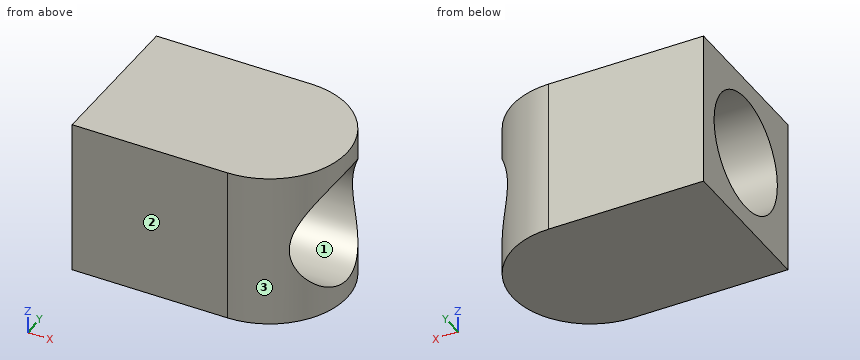
from build123d import *

# Parameters (mm, degrees)
SKETCH1_W           = 20
SKETCH1_H           = 20
BOSS_EXTRUDE1_DEPTH = 30
FILLET3_RADIUS      = 10
FILLET3_LENGTH      = 20
SKETCH2_R           = 7.5
CUT_EXTRUDE1_DEPTH  = 30


with BuildPart() as part:
    # Sketch1 → Boss-Extrude1 (new body)
    with BuildSketch(Plane(origin=(0, 0, 0), x_dir=(0, 0, -1), z_dir=(1, 0, 0))):
        Rectangle(SKETCH1_W, SKETCH1_H)
    extrude(amount=BOSS_EXTRUDE1_DEPTH)

    # Fillet3: full round fillet: the end face becomes a half cylinder, R = half its width
    fillet3_face = Plane((30, 0, 0), x_dir=(0, 0, 1), z_dir=(1, 0, 0))  # on the end face: x along it, z out of the body
    fillet3_slab = fillet3_face.offset(-FILLET3_RADIUS / 2) * Box(FILLET3_LENGTH, 2 * FILLET3_RADIUS, FILLET3_RADIUS, mode=Mode.PRIVATE)  # the body's end, R deep
    fillet3_round = Plane((20, 0, 0), x_dir=(1, 0, 0), z_dir=(0, 0, 1)) * Cylinder(FILLET3_RADIUS, FILLET3_LENGTH, mode=Mode.PRIVATE)  # its axis R under the face
    add(fillet3_slab - fillet3_round, mode=Mode.SUBTRACT)

    # Sketch2 → Cut-Extrude1 (cut)
    with BuildSketch(Plane.ZY):
        Circle(SKETCH2_R)
    extrude(amount=-CUT_EXTRUDE1_DEPTH, mode=Mode.SUBTRACT)


solid = part.part
Design review of the part built by this model. Coordinates are the model's own, in mm. Face numbers are marked on the shaded views. Coordinates: 2 decimals unless noted, no trailing zeros. Order: outer loops, then holes, each group sorted by start corner. A loop starts at its lowest first (then second) coordinate and runs counter-clockwise, first axis right, second up. Notation, with made-up numbers: (-26, -20.75) -> (2, -20.75) arc R9 cw to (2, -5.75) -> close; hole circle Ø8 at (-22.75, -12.75). An arc over 180 degrees is marked (long way). Use one line per item in the form item = value. Start each with the question number.
(1) For probe 1 along Y at (x, z) = (7.5, 0); probe 2 along Z at (x, y) = (17.5, -3.25), list the stretches that pass through material, from the lowest coordinate up.
(2) Add section C-C on x = 11. State the section outline as (y, z) points, plus the area to 3 significant figures.
(3) The part is to be moulded in two halves that separate along Y. For the marked faces 1, 2 and 3, say which applies: +Y half, -Y half, draft (parallel to the pull), parting line (faces both ways), or undercut.
(4) Add section D-D on z = 8. State the section outline as (x, y) points.
(5) Add section B-B on y = 0. State the section outline as (x, z) points.
(6) Add section A-A on z = -4.5. State the section outline as (x, y) points.
(7) Insertion check: pin 1 (10 mm diameter, centred on y = 7, z = -7.5, fed in from +X). The pin has a flat end and moves straight along its axis. Give the tip position at first contact, or say it passes through.
Answer block:
q1.probe_1 = -10 to -7.5, 7.5 to 10
q1.probe_2 = -10 to -6.76, 6.76 to 10
q2.outline = (-10, -10) -> (10, -10) -> (10, 10) -> (-10, 10) -> close; hole circle Ø15 at (0, 0)
q2.area = 223 mm²
q3.face_1 = undercut
q3.face_2 = -Y half
q3.face_3 = parting line
q4.outline = (0, -10) -> (20, -10) arc R10 ccw to (20, 10) -> (0, 10) -> close
q5.outline = (0, -10) -> (30, -10) -> (30, -7.5) -> (0, -7.5) -> close; (0, 7.5) -> (30, 7.5) -> (30, 10) -> (0, 10) -> close
q6.outline = (0, -10) -> (20, -10) arc R10 ccw to (28, -6) -> (0, -6) -> close; (0, 6) -> (28, 6) arc R10 ccw to (20, 10) -> (0, 10) -> close
q7.pin_1 = 29.8
